from build123d import *

# Parameters (mm, degrees)
CROQUIS1_W              = 164.9
CROQUIS1_H              = 102
SALIENTE_EXTRUIR1_DEPTH = 14.27
CROQUIS2_W              = 11
CROQUIS2_H              = 15
SALIENTE_EXTRUIR3_DEPTH = 6
CROQUIS3_W              = 6
CROQUIS3_H              = 7
SALIENTE_EXTRUIR4_DEPTH = 3
CROQUIS4_W              = 15
CROQUIS4_H              = 6
SALIENTE_EXTRUIR5_DEPTH = 5
SALIENTE_EXTRUIR6_DEPTH = 10
SALIENTE_EXTRUIR7_DEPTH = 4
CROQUIS7_R              = 1.5
SALIENTE_EXTRUIR8_DEPTH = 4


with BuildPart() as part:
    # Croquis1 → Saliente-Extruir1 (new body)
    with BuildSketch(Plane(origin=(0, 0, 0), x_dir=(0, 0, -1), z_dir=(1, 0, 0))):
        with Locations((10.245979532, -7.846345029)):
            Rectangle(CROQUIS1_W, CROQUIS1_H)
    extrude(amount=SALIENTE_EXTRUIR1_DEPTH)

    # Croquis2 → Saliente-Extruir3 (add)
    with BuildSketch(Plane.ZY):
        with Locations((-87.195979532, 1.653654971)):
            Rectangle(CROQUIS2_W, CROQUIS2_H)
    extrude(amount=SALIENTE_EXTRUIR3_DEPTH)

    # Croquis3 → Saliente-Extruir4 (add)
    with BuildSketch(Plane.ZY):
        with Locations((-89.695979532, -36.846345029)):
            Rectangle(CROQUIS3_W, CROQUIS3_H)
        with Locations((-89.695979532, -18.846345029)):
            Rectangle(CROQUIS3_W, CROQUIS3_H)
    extrude(amount=SALIENTE_EXTRUIR4_DEPTH)

    # Croquis4 → Saliente-Extruir5 (add)
    with BuildSketch(Plane.ZY):
        with Locations((64.704020468, -35.686345029)):
            Rectangle(CROQUIS4_W, CROQUIS4_H)
    extrude(amount=SALIENTE_EXTRUIR5_DEPTH)

    # Croquis5 → Saliente-Extruir6 (add)
    with BuildSketch(Plane.ZY):
        with BuildLine():
            Line((-80.945979532, 40.553654971), (-50.445979532, 40.553654971))
            ThreePointArc((-50.445979532, 40.553654971), (-46.910445626, 39.089188877), (-45.445979532, 35.553654971))
            Line((-45.445979532, 35.553654971), (-45.445979532, 16.753654971))
            ThreePointArc((-45.445979532, 16.753654971), (-46.910445626, 13.218121065), (-50.445979532, 11.753654971))
            Line((-50.445979532, 11.753654971), (-80.945979532, 11.753654971))
            ThreePointArc((-80.945979532, 11.753654971), (-84.481513438, 13.218121065), (-85.945979532, 16.753654971))
            Line((-85.945979532, 16.753654971), (-85.945979532, 35.553654971))
            ThreePointArc((-85.945979532, 35.553654971), (-84.481513438, 39.089188877), (-80.945979532, 40.553654971))
        make_face()
        with BuildLine():
            Line((29.954020468, 40.553654971), (60.454020468, 40.553654971))
            ThreePointArc((60.454020468, 40.553654971), (63.989554374, 39.089188877), (65.454020468, 35.553654971))
            Line((65.454020468, 35.553654971), (65.454020468, 16.753654971))
            ThreePointArc((65.454020468, 16.753654971), (63.989554374, 13.218121065), (60.454020468, 11.753654971))
            Line((60.454020468, 11.753654971), (29.954020468, 11.753654971))
            ThreePointArc((29.954020468, 11.753654971), (26.418486562, 13.218121065), (24.954020468, 16.753654971))
            Line((24.954020468, 16.753654971), (24.954020468, 35.553654971))
            ThreePointArc((24.954020468, 35.553654971), (26.418486562, 39.089188877), (29.954020468, 40.553654971))
        make_face()
    extrude(amount=SALIENTE_EXTRUIR6_DEPTH)

    # Croquis6 → Saliente-Extruir7 (add)
    with BuildSketch(Plane.ZY):
        with BuildLine():
            Line((58.204020468, -2.846345029), (65.204020468, -2.846345029))
            ThreePointArc((65.204020468, -2.846345029), (70.153767936, -4.896597561), (72.204020468, -9.846345029))
            Line((72.204020468, -9.846345029), (72.204020468, -11.846345029))
            ThreePointArc((72.204020468, -11.846345029), (70.153767936, -16.796092498), (65.204020468, -18.846345029))
            Line((65.204020468, -18.846345029), (58.204020468, -18.846345029))
            Line((58.204020468, -18.846345029), (58.204020468, -2.846345029))
        make_face()
    extrude(amount=SALIENTE_EXTRUIR7_DEPTH)

    # Croquis7 → Saliente-Extruir8 (add)
    with BuildSketch(Plane.ZY):
        with Locations(Location((-87.690979532, 38.153654971, 0), (0, 0, 180))):
            Circle(CROQUIS7_R)
        with Locations(Location((67.204020468, 38.153654971, 0), (0, 0, 180))):
            Circle(CROQUIS7_R)
        with Locations(Location((-87.695979532, -53.846345029, 0), (0, 0, 180))):
            Circle(CROQUIS7_R)
        with Locations(Location((67.204020468, -53.846345029, 0), (0, 0, 180))):
            Circle(CROQUIS7_R)
    extrude(amount=SALIENTE_EXTRUIR8_DEPTH)


solid = part.part
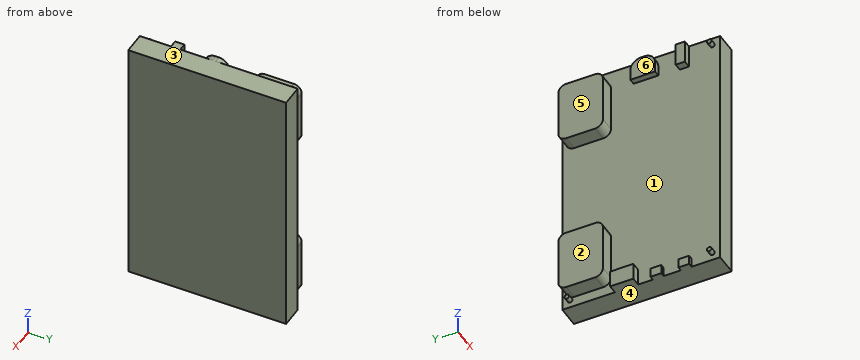
Can you work these out from the model? Positions are in its coordinate system, mm. Face numbers are marked on the shaded views. A direction names the side the tool comes from. Coordinates: 2 decimals unless noted, no trailing zeros. Write each loop counter-clockwise with the first axis right and the second up, starting at its lowest first coordinate (ties: lowest second). Pieces come first, ordered by that corner, then holes. Notation, with made-up numbers: (-13, 50) -> (-6, 50) arc R22 ccw to (-6, 58) -> close; hole circle Ø4 at (22.5, 35). An arc over 180 degrees is marked (long way). Write each question's results on one line, items separated by ' | '. Start each with the question number.
Item 1: If we section it at C-C, the plane z = -11: Write out the boundary of the cut face in (x, y).
Item 2: If we section it at B-B, the plane z = 35.5: Write out the boundary of the cut face in (x, y).
Item 3: I'm going to push flat-ended pins straight in: P1, Ø6, axis at y = -4, z = -4.5, coming from the -X side; P2, Ø5, axis at x = -4.5, z = -60, coming from the +Y side; P3, Ø3.5, axis at y = 38.5, z = 67.5, coming from the -X side. Where does each tip first touch, or does it pass through?
Item 4: On a 3-axis mill with a long thin cutter (end or side, diameter ignored), from which of +Z, -Z, +X, -X, +Y, -Y can I reach the whole of each face in a straight line? I mean the marked faces 5 and 6. Say none if no direction works.
Item 5: If we section it at A-A, the plane y = 33.5: Write out the boundary of the cut face in (x, z), and give its area (3 significant figures).
Item 6: Thinking about a two-plate mould opening in Z: for the marked faces 1, 2, 3 and 4, which applies, released by +Z, released by -Z, zero draft, split by the parting line, or undercut?
Item 7: Please list where these lines run through material, in increasing order: probe 1 along Z at (x, y) = (-1.75, -36); probe 2 along X at (y, z) = (-1, -35.5); probe 3 along Z at (x, y) = (-1.5, 16.5).
Answer block:
1) outline: (0, -58.85) -> (14.27, -58.85) -> (14.27, 43.15) -> (0, 43.15) -> close
2) outline: (-10, 11.75) -> (0, 11.75) -> (0, -58.85) -> (14.27, -58.85) -> (14.27, 43.15) -> (0, 43.15) -> (0, 40.55) -> (-10, 40.55) -> close
3) P1: x = 0 | P2: y = 40.55 | P3: x = -4
4) face 5: +Z, -Z, -X, +Y, -Y | face 6: +Z, -X
5) outline: (-10, -85.95) -> (0, -85.95) -> (0, -92.7) -> (14.27, -92.7) -> (14.27, 72.2) -> (0, 72.2) -> (0, 65.45) -> (-10, 65.45) -> (-10, 24.95) -> (0, 24.95) -> (0, -45.45) -> (-10, -45.45) -> close | area: 3,160 mm²
6) face 1: undercut | face 2: zero draft | face 3: released by +Z | face 4: released by -Z
7) probe 1: -92.7 to -86.7, 57.2 to 72.2 | probe 2: 0 to 14.27 | probe 3: -85.94 to -45.45, 24.96 to 65.45
